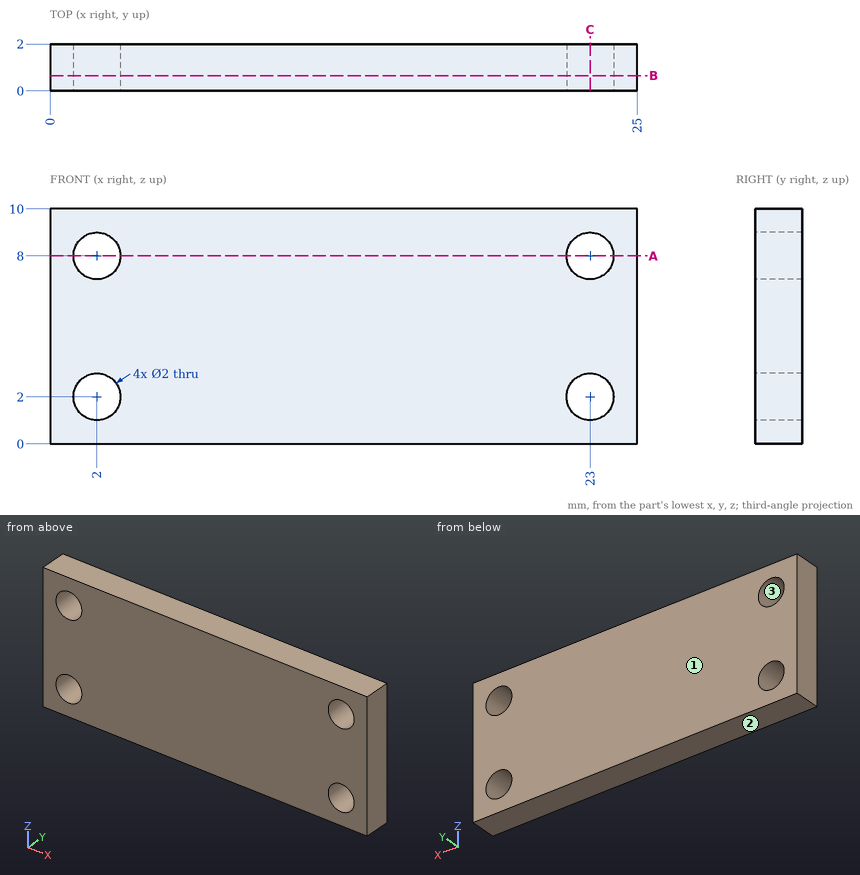
Geometry check sheet. Reference: drawing and pictorial views, mm from the part's lowest x, y, z. Round coordinates to 2 decimals unless told otherwise and drop trailing zeros. Loops run counter-clockwise (first coordinate to the right, second up) from the corner with the lowest first, then second, coordinate; pieces in that order, holes last. Notation, with made-up numbers: M -26,-19.5 L 10,-19.5 A14 cw 10,-5.5 Z; hole C 31.5,53.5 d2. An arc over 180 degrees is marked long. Return JSON: item names as keys, results as strings. Group by question number.
(1) Go/stop test with a flat-tipped pin: pin 1 (3 mm diameter, centred on x = 23, z = 2, fed in from +Y). Record where the tip stops, or that it passes through.
(2) Section check B-B, the plane y = 0.65. Enter the section's corners in (x, z).
(3) Section check C-C, the plane x = 23. Enter the section's corners in (y, z), and give its area (3 significant figures).
(4) Section check A-A, the plane z = 8. Enter the section's corners in (x, y), and give its area (3 significant figures).
(5) Mould release check, pull along Z, two halves, no side actions. Record for the marked faces 1, 2 and 3: pulls with the +Z half, pulls with the -Z half, needs draft (parallel to the pull), parting line crosses it, or undercut.
(6) Scan lines: line 1 along Z through (x, y) = (2, 1.6); line 2 along X through (y, z) = (0.9, 1.5); line 3 along Z through (x, y) = (23.75, 1.2). Record each from-to range of solid material in increasing order. Write a range as [from, to].
Data:
{
 "1": {"pin 1": "y = 2"},
 "2": {"outline": "M 0,0 L 25,0 L 25,10 L 0,10 Z; hole C 2,2 d2; hole C 2,8 d2; hole C 23,2 d2; hole C 23,8 d2"},
 "3": {"outline": "M 0,0 L 2,0 L 2,1 L 0,1 Z; M 0,3 L 2,3 L 2,7 L 0,7 Z; M 0,9 L 2,9 L 2,10 L 0,10 Z", "area": "12.0 mm²"},
 "4": {"outline": "M 0,0 L 1,0 L 1,2 L 0,2 Z; M 3,0 L 22,0 L 22,2 L 3,2 Z; M 24,0 L 25,0 L 25,2 L 24,2 Z", "area": "42.0 mm²"},
 "5": {"face 1": "needs draft", "face 2": "pulls with the -Z half", "face 3": "undercut"},
 "6": {"line 1": "[0, 1], [3, 7], [9, 10]", "line 2": "[0, 1.13], [2.87, 22.13], [23.87, 25]", "line 3": "[0, 1.34], [2.66, 7.34], [8.66, 10]"}
}
